Source: CAD feature listing. Evaluate the final solid. Frame: model axes, mm. A direction names the side the tool comes from. Give positions to 0.01 mm unless a question says otherwise; leave off trailing zeros. Write each loop counter-clockwise with the first axis right and the second up, starting at its lowest first coordinate (ties: lowest second). Pieces come first, ordered by that corner, then holes. Notation, with made-up numbers: M -24,-36.5 L -5,-36.5 A16 cw -5,-20.5 Z; hole C 14,-21 d9. An arc over 180 degrees is marked long. Return JSON: item names as keys, results as strings.
```python
from build123d import *

# Parameters (mm, degrees)
SKETCH1_R           = 254
SKETCH1_R_2         = 233.4
BOSS_EXTRUDE1_DEPTH = 2250
SKETCH2_R           = 57.25
CUT_EXTRUDE1_DEPTH  = 2250
SKETCH3_R           = 57.25
SKETCH3_R_2         = 24.5
CUT_EXTRUDE2_DEPTH  = 2250


with BuildPart() as part:
    # Sketch1 → Boss-Extrude1 (new body)
    with BuildSketch(Plane.XY):
        Circle(SKETCH1_R)
        Circle(SKETCH1_R_2, mode=Mode.SUBTRACT)
    extrude(amount=-BOSS_EXTRUDE1_DEPTH)

    # Sketch2 → Cut-Extrude1 (cut)
    with BuildSketch(Plane(origin=(0, 0, 0), x_dir=(1, 0, 0), z_dir=(0, 1, 0))):
        with Locations(Location((0, 179, 0), (0, 0, 90))):
            Circle(SKETCH2_R)
    extrude(amount=CUT_EXTRUDE1_DEPTH, mode=Mode.SUBTRACT)

    # Sketch3 → Cut-Extrude2 (cut)
    with BuildSketch(Plane(origin=(0, 0, 0), x_dir=(1, 0, 0), z_dir=(0, 1, 0))):
        with Locations(Location((0, 2049, 0), (0, 0, 270))):
            Circle(SKETCH3_R)
        with Locations(Location((0, 649, 0), (0, 0, 270))):
            Circle(SKETCH3_R_2)
    extrude(amount=-CUT_EXTRUDE2_DEPTH, mode=Mode.SUBTRACT)


solid = part.part
```
1) Line query: line 1 (Z direction, x = 0, y = -249); line 2 (Y direction, x = 0, z = -755.5); line 3 (X direction, y = 8, z = -1129). Output: solid intervals per line, ascending. Write a range as [from, to].
Numbers:
{"line 1": "z = [-2250, -2106.25], [-1991.75, -673.5], [-624.5, 0]", "line 2": "y = [-254, -233.4], [233.4, 254]", "line 3": "x = [-253.87, -233.26], [233.26, 253.87]"}
2) Draft query along X for faces 1 (the face through (-55.06, -247.96, -1109.25)), 2 (the face through (56.763, -239.941, -2056.453)), 3 (the face through (206, -112, -2250)). Return one class per face: released by +X, released by -X, zero draft, split by the parting line, or undercut.
Numbers:
{"face 1": "split by the parting line", "face 2": "undercut", "face 3": "zero draft"}
3) Contact query for flat-ended pins moving along their axis: pin 1 Ø5 at (y, z) = (-34, -431) entering from -X; pin 2 Ø1.5 at (x, z) = (180.5, -854) entering from -Y; pin 3 Ø3 at (y, z) = (21, -1171.5) entering from -X. Output: stop coordinate, or through.
Numbers:
{"pin 1": "stops at x = -252.04", "pin 2": "stops at y = -179.46", "pin 3": "stops at x = -253.25"}
4) Cut plane B-B, the plane y = 0. Return the cut outline in (x, z).
Numbers:
{"outline": "M -254,-2250 L -233.4,-2250 L -233.4,0 L -254,0 Z; M 233.4,-2250 L 254,-2250 L 254,0 L 233.4,0 Z"}
5) Cut plane A-A, the plane x = 0. Return the cut outline in (y, z), then the cut area to 3 significant figures.
Numbers:
{"outline": "M -254,-2250 L -233.4,-2250 L -233.4,-2106.25 L -254,-2106.25 Z; M -254,-1991.75 L -233.4,-1991.75 L -233.4,-673.5 L -254,-673.5 Z; M -254,-624.5 L -233.4,-624.5 L -233.4,0 L -254,0 Z; M 233.4,-2250 L 254,-2250 L 254,-236.25 L 233.4,-236.25 Z; M 233.4,-121.75 L 254,-121.75 L 254,0 L 233.4,0 Z", "area": "87,000 mm²"}
6) Cut plane D-D, the plane z = -974. Return the cut outline in (x, y).
Numbers:
{"outline": "C 0,0 d508; hole C 0,0 d466.8"}
7) Set-up query: faces 4 (the face through (1.077, -242.903, -673.476)), 5 (the face through (-56.763, 239.941, -171.547)), 6 (the face through (206, -112, 0)). Return all of +Z, -Z, +X, -X, +Y, -Y with unobstructed straight access to the full face (end or side cutting, diameter ignored); none if empty.
Numbers:
{"face 4": "-Y", "face 5": "+Y", "face 6": "+Z, +X, -X, +Y, -Y"}
8) Cut plane C-C, the plane x = -131.5. Return the cut outline in (y, z).
Numbers:
{"outline": "M -217.31,-2250 L -192.83,-2250 L -192.83,0 L -217.31,0 Z; M 192.83,-2250 L 217.31,-2250 L 217.31,0 L 192.83,0 Z"}
